```python
from build123d import *

# Parameters (mm, degrees)
F0_R     = 1.27
F1_DEPTH = 12.7
F3_D     = 15.875
F6_D     = 12.7
F8_D     = 12.7


# Not quite as in the source:
# - a feature names something its author has since deleted; it is built from what else it names


with BuildPart() as f1:
    # F0 (on Top) → F1 (new body)
    with BuildSketch(Plane.XY):
        Polygon((200.6098739386, 63.1592117809), (-2.5901260614, 63.1592117809), (-104.1901260614, 63.1592117809), (-104.1901260614, -38.4407882191), (-2.5901260614, -38.4407882191), (200.6098739386, -38.4407882191), align=None)
        with Locations((-53.3901260614, -19.3907882191)):
            Circle(F0_R, mode=Mode.SUBTRACT)
        with Locations((-78.4163327398, -7.1792497576)):
            Circle(F0_R, mode=Mode.SUBTRACT)
        with Locations((-53.3901260614, 12.3592117809)):
            Circle(F0_R, mode=Mode.SUBTRACT)
        with Locations((-23.1804483045, 2.5899810116)):
            Circle(F0_R, mode=Mode.SUBTRACT)
        with Locations((-85.1401260614, 12.3592117809)):
            Circle(F0_R, mode=Mode.SUBTRACT)
        with Locations((-92.6627071454, 25.0592117809)):
            Circle(F0_R, mode=Mode.SUBTRACT)
        with Locations((-12.1151260614, 12.3592117809)):
            Circle(F0_R, mode=Mode.SUBTRACT)
        with Locations((-20.8560573795, 37.7592117809)):
            Circle(F0_R, mode=Mode.SUBTRACT)
        with Locations((-53.3901260614, 53.6342117809)):
            Circle(F0_R, mode=Mode.SUBTRACT)
        with Locations((-92.6627071454, 25.0592117809)):
            Circle(F0_R)
        with Locations((-53.3901260614, 53.6342117809)):
            Circle(F0_R)
        with Locations((-20.8560573795, 37.7592117809)):
            Circle(F0_R)
        with Locations((-12.1151260614, 12.3592117809)):
            Circle(F0_R)
    extrude(amount=F1_DEPTH)

    # F3 (through all)
    with Locations(Plane.XY.offset(12.7)):
        with Locations((-53.3901260614, 12.3592117809)):
            Hole(F3_D / 2)

    # F6 (through all)
    with Locations(Plane.XY.offset(12.7)):
        with Locations((-53.3901260614, -19.3907882191)):
            Hole(F6_D / 2)

    # F8 (through all)
    with Locations(Plane.XY.offset(12.7)):
        with Locations((-85.1401260614, 12.3592117809), (-78.4163327398, -7.1792497576), (-23.1804483045, 2.5899810116)):
            Hole(F8_D / 2)


solid = f1.part
```
Here's how the part is built. I have some questions about the finished solid (model axes, mm). Coordinates: 2 decimals unless noted, no trailing zeros. Use a Markdown table: item, result. Add a question column.
(1) Please list where these lines run through material, in increasing order: line 1 (X direction, y = -7, z = 9.5); line 2 (X direction, y = 16, z = 4.5); line 3 (Y direction, x = -88, z = 5.25).
(2) If we section it at A-A, the plane z = 5.25: State how many separate pieces and enclosed holes the cut face has, and give its area (3 significant figures).
(3) We'd pull the mould along Y, two halves only. Please class faces 1 (the flat face through (50, 63.159, 6)), 2 (the flat face through (46, -38.441, 6)), 3 (the cylindrical face through (-59.256, -21.823, 6.261)): +Y half, -Y half, draft (parallel to the pull), parting line (faces both ways), or undercut.
(4) I'm going to push flat-ended pins straight in: P1, Ø20.5, axis at x = -23.18, y = 2.59, coming from the -Z side; P2, Ø10, axis at x = -85.14, y = 12.36, coming from the +Z side. Where does each tip first touch, or does it pass through?
Outcome:
| question | item | result |
|---|---|---|
| 1 | line 1 | x = -104.19 to -84.76, -72.07 to 200.61 |
| 1 | line 2 | x = -104.19 to -90.34, -79.94 to -60.44, -46.34 to 200.61 |
| 1 | line 3 | y = -38.44 to 6.69, 18.03 to 63.16 |
| 2 | separate pieces | 1 |
| 2 | enclosed holes | 5 |
| 2 | area | 30,300 mm^2 |
| 3 | face 1 | +Y half |
| 3 | face 2 | -Y half |
| 3 | face 3 | undercut |
| 4 | P1 | stops at z = 0 |
| 4 | P2 | passes through |
